Model file for the job. Use its own axes, mm. A direction names the side the tool comes from. Give positions to 0.01 mm unless a question says otherwise; leave off trailing zeros. Write each loop counter-clockwise with the first axis right and the second up, starting at its lowest first coordinate (ties: lowest second). Pieces come first, ordered by that corner, then holes. Notation, with made-up numbers: (30, -3) - (50, -3) arc R16 ccw to (50, 4) - close; hole circle Ø11 at (67.25, 48.25). An arc over 180 degrees is marked (long way). Use CSV: the item, a comma, the result in double quotes.
from build123d import *

# Parameters (mm, degrees)
F0_W     = 80
F0_H     = 50
F1_DEPTH = 50
F2_R     = 10
F3_T     = -2.5
F5_D     = 5
F5_DEPTH = 12
F6_W     = 8.087612
F6_H     = 4.312344
F7_DEPTH = 25


with BuildPart() as f1:
    # F0 (on Front) → F1 (new body)
    with BuildSketch(Plane.XZ):
        Rectangle(F0_W, F0_H)
    extrude(amount=F1_DEPTH)

    # F2
    f2_edges = [f1.edges().sort_by_distance(p)[0] for p in [
        (40, -25, -25),
        (-40, -25, -25),
        (40, 0, 0),
        (0, 0, -25),
        (-40, 0, 0),
    ]]
    fillet(f2_edges, radius=F2_R)

    # F3
    f3_openings = [f1.faces().sort_by_distance(p)[0] for p in [
        (0, -50, 0.246934),
    ]]
    offset(amount=F3_T, openings=f3_openings)

    # F5
    with Locations(Plane(origin=(0, 0, -25), x_dir=(1, 0, 0), z_dir=(0, 0, -1))):
        with Locations((-10, 20)):
            Hole(F5_D / 2, depth=F5_DEPTH)

    # F6 (on face) → F7 (cut)
    with BuildSketch(Plane.YZ.offset(40)):
        with Locations((-45.956194, 19.277418)):
            Rectangle(F6_W, F6_H)
    extrude(amount=-F7_DEPTH, mode=Mode.SUBTRACT)


solid = f1.part
(1) Flat gauge pins, fed straight in: P1, Ø6, axis at x = 26, y = -6.5, coming from the -Z side; P2, Ø4.5, axis at x = -10, y = -20, coming from the -Z side; P3, Ø1, axis at x = -8.5, z = 1.5, coming from the -Y side. Where does each tip first touch, or does it go through?
Checked values:
P1,"stops at z = -24.99"
P2,"stops at z = 22.5"
P3,"stops at y = -2.5"
(2) Saw through at D-D, the plane y = -20. List the corners of the cut face in (x, z), then the cut area to 3 significant figures.
Checked values:
outline,"(-40, -15) arc R10 ccw to (-30, -25) - (-12.5, -25) - (-12.5, -22.5) - (-30, -22.5) arc R7.5 cw to (-37.5, -15) - (-37.5, 22.5) - (37.5, 22.5) - (37.5, -15) arc R7.5 cw to (30, -22.5) - (-7.5, -22.5) - (-7.5, -25) - (30, -25) arc R10 ccw to (40, -15) - (40, 25) - (-40, 25) - close"
area,"594 mm^2"
(3) Saw through at A-A, the plane x = -11.5. List the corners of the cut face in (y, z), then the cut area to 3 significant figures.
Checked values:
outline,"(-50, -25) - (-22, -25) - (-22, -22.5) - (-50, -22.5) - close; (-50, 22.5) - (-2.5, 22.5) - (-2.5, -15) arc R7.5 cw to (-10, -22.5) - (-18, -22.5) - (-18, -25) - (-10, -25) arc R10 ccw to (0, -15) - (0, 25) - (-50, 25) - close"
area,"343 mm^2"
(4) Pull direction Z, two halves, no side cores. Call faces 4 (the face through (40, -30, 5)), 5 (the face through (39, -41.912, 19)), 6 (the face through (36.99, -30.28, -22.15)): released by +Z, released by -Z, zero draft, split by the parting line, or undercut.
Checked values:
face 4,"zero draft"
face 5,"undercut"
face 6,"released by -Z"
(5) Wall check: probe 1 along Z at (x, y) = (30, -45.5); probe 2 along X at (y, z) = (-27, 9); probe 3 along Y at (x, z) = (-19, -2.5). Give the ranges that are in metal, low to high. Write a range as [from, to].
Checked values:
probe 1,"z = [-25, -22.5], [22.5, 25]"
probe 2,"x = [-40, -37.5], [37.5, 40]"
probe 3,"y = [-2.5, 0]"
(6) 3-axis set-ups, long thin cutter, end or side, ignore diameter. For faces 1 (the face through (39, -46, 21.434)), 2 (the face through (-40, -30, 5)), 3 (the face through (-1, -26, 22.5)): which of +Z, -Z, +X, -X, +Y, -Y reach the whole face in a straight line?
Checked values:
face 1,"+X, -Y"
face 2,"+Z, -Z, -X, +Y, -Y"
face 3,"-Y"
(7) Saw through at B-B, the plane y = -30.5. List the corners of the cut face in (x, z).
Checked values:
outline,"(-40, -15) arc R10 ccw to (-30, -25) - (30, -25) arc R10 ccw to (40, -15) - (40, 25) - (-40, 25) - close; hole (-37.5, -15) arc R7.5 ccw to (-30, -22.5) - (30, -22.5) arc R7.5 ccw to (37.5, -15) - (37.5, 22.5) - (-37.5, 22.5) - close"
(8) Saw through at C-C, the plane z = -13.5. List the corners of the cut face in (x, y), then the cut area to 3 significant figures.
Checked values:
outline,"(-40, -50) - (-37.5, -50) - (-37.5, -10) arc R7.5 cw to (-30, -2.5) - (30, -2.5) arc R7.5 cw to (37.5, -10) - (37.5, -50) - (40, -50) - (40, -10) arc R10 ccw to (30, 0) - (-30, 0) arc R10 ccw to (-40, -10) - close"
area,"419 mm^2"
